Source: CAD feature listing. Evaluate the final solid. Frame: model axes, mm. Give positions to 0.01 mm unless a question says otherwise; leave off trailing zeros. Write each loop counter-clockwise with the first axis right and the second up, starting at its lowest first coordinate (ties: lowest second). Pieces come first, ordered by that corner, then holes. Notation, with made-up numbers: (-4.75, 14) - (40.25, 14) arc R13 ccw to (40.25, 27) - close; hole circle Ø10 at (-10.75, 36.25). An arc over 180 degrees is marked (long way). Answer as a JSON object with one key per item and string values. Group by question number.
from build123d import *

# Parameters (mm, degrees)
F0_R     = 37.5
F0_R_2   = 11
F1_DEPTH = 3.5


# Not quite as in the source:
# - a pattern or mirror of a feature is missing from the dataset's text; its kind, count and spacing are read off the source's solid


with BuildPart() as f1:
    # F0 (on Top) → F1 (new body, symmetric)
    with BuildSketch(Plane.XY):
        Circle(F0_R)
        Circle(F0_R_2, mode=Mode.SUBTRACT)
    extrude(amount=F1_DEPTH, both=True)

    # F2 (on Right) → F3 (revolve, cut)
    with BuildSketch(Plane.YZ):
        Polygon((43.8578222282, 0.5), (43.8578222282, 0), (53.1842447817, 0), (53.1842447817, 16.8883297592), (14, 16.8883297592), (14, 3.5), align=None)
    f3 = revolve(axis=Axis((0, 0, 12.1004180983), (0, 0, 1)), mode=Mode.SUBTRACT)

    # F3_copies: F3 across plane
    add(f3.mirror(Plane(origin=(0, 0, 0), x_dir=(-1, 0, 0), z_dir=(0, 0, -1))), mode=Mode.SUBTRACT)


solid = f1.part
Q1. Section C-C on z = 2. Return the cut outline in (x, y).
Q2. Section A-A on y = 0. Return the cut outline in (x, z).
Q3. Ray query, probe 1 along Y at (x, z) = (0, 1); probe 2 along X at (y, z) = (0.5, 0.5); probe 3 along X at (y, z) = (6, -0.75). Return the intervals inside material, ascending. Write a range as [from, to].
Q4. First-contact query: pin 1 Ø4 at (x, y) = (24.5, 9.5) entering from +Z; pin 2 Ø1 at (y, z) = (1.5, -0.5) entering from +X; pin 3 Ø3 at (x, z) = (3, -2) entering from -Y; pin 4 Ø17.5 at (x, y) = (0, 0) entering from +Z. Flat tips, straight axial feed; report the tip coordinate or a pass-through.
Q5. Draft query along X for faces 1 (the flat face through (6.2, -9.3, 3.5)), 2 (the conical face through (-4.65, 14.76, 3.35)), 3 (the cylindrical face through (-2.38, -10.74, -0.05)). Return one class per face: released by +X, released by -X, zero draft, split by the parting line, or undercut.
Taken from the geometry:
{
 "1": {"outline": "circle Ø57.86 at (0, 0); hole circle Ø22 at (0, 0)"},
 "2": {"outline": "(-37.5, -1.14) - (-14, -3.5) - (-11, -3.5) - (-11, 3.5) - (-14, 3.5) - (-37.5, 1.14) - close; (11, -3.5) - (14, -3.5) - (37.5, -1.14) - (37.5, 1.14) - (14, 3.5) - (11, 3.5) - close"},
 "3": {"probe 1": "y = [-37.5, -11], [11, 37.5]", "probe 2": "x = [-37.5, -10.99], [10.99, 37.5]", "probe 3": "x = [-37.02, -9.22], [9.22, 37.02]"},
 "4": {"pin 1": "stops at z = 2.47", "pin 2": "stops at x = 37.49", "pin 3": "stops at y = -37.46", "pin 4": "passes through"},
 "5": {"face 1": "zero draft", "face 2": "split by the parting line", "face 3": "undercut"}
}
